from build123d import *

# Parameters (mm, degrees)
BOSS_EXTRU_1_DEPTH                                 = 22
ESQUISSE2_W                                        = 22
ESQUISSE2_H                                        = 6
BOSS_EXTRU_2_DEPTH                                 = 5
CHAMBRAGE_POUR_VIS_T_TE_HEXAGONALE_M21_D           = 2
CHAMBRAGE_POUR_VIS_T_TE_HEXAGONALE_M21_CBORE_D     = 4
CHAMBRAGE_POUR_VIS_T_TE_HEXAGONALE_M21_CBORE_DEPTH = 2
CONG_1_R                                           = 10
CONG_2_R                                           = 1


# Some blends are built 0.0001 mm under size
with BuildPart() as part:
    # Esquisse1 → Boss.-Extru.1 (new body)
    with BuildSketch(Plane.XY):
        with BuildLine():
            Line((0, 6), (0, 0))
            Line((0, 0), (6, 0))
            ThreePointArc((6, 0), (11, 5), (16, 0))
            Line((16, 0), (22, 0))
            Line((22, 0), (22, 6))
            Line((22, 6), (0, 6))
        make_face()
    extrude(amount=BOSS_EXTRU_1_DEPTH)

    # Esquisse2 → Boss.-Extru.2 (add)
    with BuildSketch(Plane.XY.offset(22)):
        with Locations((11, 3)):
            Rectangle(ESQUISSE2_W, ESQUISSE2_H)
    extrude(amount=BOSS_EXTRU_2_DEPTH)

    # Chambrage pour vis à tête hexagonale M21 (through all)
    with Locations(Plane(origin=(0, 6, 0), x_dir=(1, 0, 0), z_dir=(0, 1, 0))):
        with Locations((19, -12), (3, -12)):
            CounterBoreHole(CHAMBRAGE_POUR_VIS_T_TE_HEXAGONALE_M21_D / 2, CHAMBRAGE_POUR_VIS_T_TE_HEXAGONALE_M21_CBORE_D / 2, CHAMBRAGE_POUR_VIS_T_TE_HEXAGONALE_M21_CBORE_DEPTH)

    # Congé1
    # the kernel refuses this fillet: 10 mm, written as the material it takes off along each edge
    with BuildSketch(Plane(origin=(0, 31, 0), x_dir=(0, 0, 1), z_dir=(0, -1, 0)), Plane(origin=(22, -25, 27), x_dir=(-1, 0, 0), z_dir=(0, 1, 0))) as cong_1_piece_1:
        with BuildLine():
            CenterArc((CONG_1_R, -CONG_1_R), CONG_1_R, 90, 90)
            Line((0, -CONG_1_R), (0, 0))
            Line((0, 0), (CONG_1_R, 0))
        make_face()
    extrude(amount=56, mode=Mode.SUBTRACT)
    with BuildSketch(Plane(origin=(0, 31, 27), x_dir=(0, 0, -1), z_dir=(0, -1, 0)), Plane(origin=(22, -25, 0), x_dir=(-1, 0, 0), z_dir=(0, 1, 0))) as cong_1_piece_2:
        with BuildLine():
            CenterArc((CONG_1_R, CONG_1_R), CONG_1_R, 180, 90)
            Line((0, CONG_1_R), (0, 0))
            Line((0, 0), (CONG_1_R, 0))
        make_face()
    extrude(amount=56, mode=Mode.SUBTRACT)

    # Congé2
    cong_2_edges = [part.edges().sort_by_distance(p)[0] for p in [
        (11, 6, 0),
        (0, 6, 13.5),
        (11, 6, 27),
        (22, 6, 13.5),
        (19.071067812, 6, 24.071067812),
        (19.071067812, 6, 2.928932188),
        (2.928932188, 6, 24.071067812),
        (2.928932188, 6, 2.928932188),
    ]]
    fillet(cong_2_edges, radius=CONG_2_R - 0.0001)  # a hair under: the kernel refuses the full size


solid = part.part
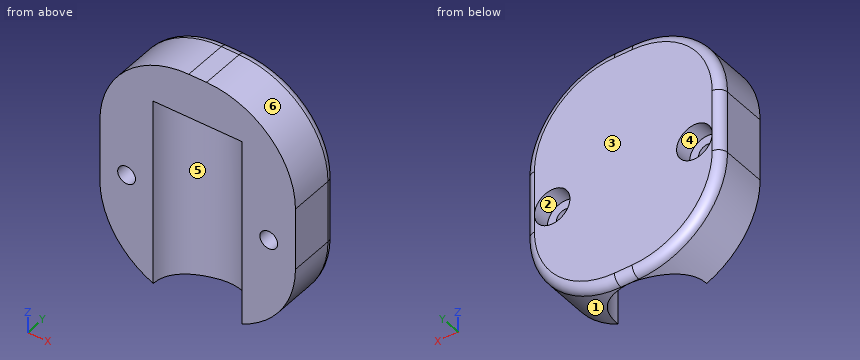
Read the model definition and answer for the solid it produces. Units are mm, in the model's axes. Face numbers are marked on the shaded views. A direction names the side the tool comes from. Give positions to 0.01 mm unless a question says otherwise; leave off trailing zeros. Loops run counter-clockwise (first coordinate to the right, second up) from the corner with the lowest first, then second, coordinate; pieces in that order, holes last. Notation, with made-up numbers: (-7.75, -22.75) - (-2.75, -22.75) arc R26 cw to (-2.75, -2.75) - close; hole circle Ø11 at (-29.75, 76.5). An arc over 180 degrees is marked (long way). Answer as CSV lines item,"result". Start each with the question number.
1) Find section D-D (z = 16). Write down the section's boundary in (x, y).
2) Determine the mould class of the marked faces 1, 2, 3 and 4 for opening direction X: released by +X, released by -X, zero draft, split by the parting line, or undercut.
3) Find section A-A (z = 12). State how many separate pieces and enclosed holes the cut face has, then the cut area to 3 significant figures.
4) Straight lines are drawn through the part: L1, parallel to X at y = 5.4, z = 12; L2, parallel to X at y = 1, z = 7.75; L3, parallel to X at y = 4.5, z = 3.5. For each, find the intervals that lie inside material, in ascending order. Write a range as from..to.
5) Each of these flat-tipped pins is pushed along its axis until it touches: pin 1 Ø1.5 at (y, z) = (2.5, 18.5) entering from +X; pin 2 Ø2.5 at (x, z) = (3, 12) entering from +Y; pin 3 Ø1.5 at (x, y) = (11, 1.5) entering from -Z. Where does it stop, or does it pass through?
6) Which of the six approach directions +Z, -Z, +X, -X, +Y, -Y give full straight-line access (tool end or side, diameter ignored) to the marked faces 5 and 6?
7) Find section C-C (y = 1). Write down the section's boundary in (x, z), then the cut area to 3 significant figures.
Findings below:
1,outline,"(0, 0) - (6, 0) arc R5 cw to (16, 0) - (22, 0) - (22, 5) arc R1 ccw to (21, 6) - (1, 6) arc R1 ccw to (0, 5) - close"
2,face 1,"released by +X"
2,face 2,"undercut"
2,face 3,"zero draft"
2,face 4,"undercut"
3,separate pieces,"3"
3,enclosed holes,"0"
3,area,"60.3 mm^2"
4,L1,"0.08..1, 5..17, 21..21.92"
4,L2,"0.26..6.1, 15.9..21.74"
4,L3,"2.4..8.82, 13.18..19.6"
5,pin 1,"x = 21.97"
5,pin 2,"y = 4"
5,pin 3,"z = 22"
6,face 5,"-Z, -Y"
6,face 6,"+Z, +X, +Y, -Y"
7,outline,"(0, 10) arc R10 ccw to (6.1, 0.79) - (6.1, 22) - (15.9, 22) - (15.9, 0.79) arc R10 ccw to (22, 10) - (22, 17) arc R10 ccw to (12, 27) - (10, 27) arc R10 ccw to (0, 17) - close; hole circle Ø2 at (3, 12); hole circle Ø2 at (19, 12)"
7,area,"288 mm^2"
